Study the drawing (mm; zero at the part's minimum x, y, z) and answer. A direction names the side the tool comes from. Coordinates: 2 decimals unless noted, no trailing zeros. Order: outer loops, then holes, each group sorted by start corner. A loop starts at its lowest first (then second) coordinate and runs counter-clockwise, first axis right, second up.
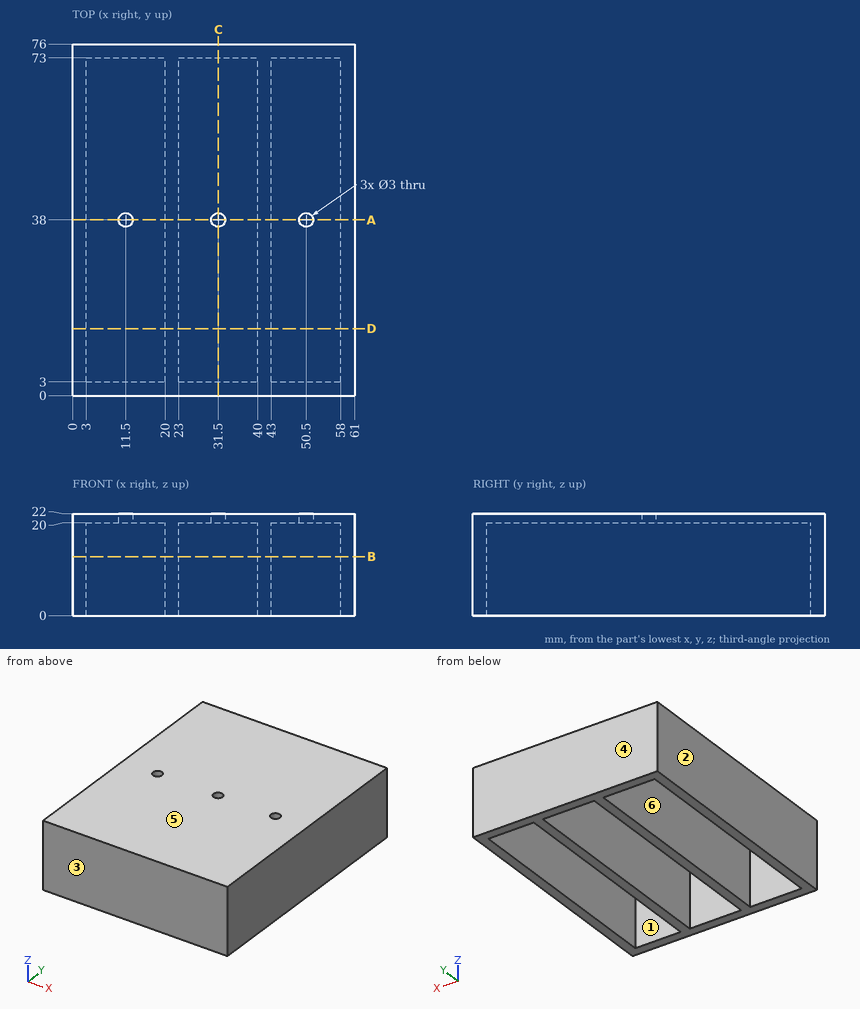
1) Which of the six approach directions +Z, -Z, +X, -X, +Y, -Y give full straight-line access (tool end or side, diameter ignored) to the marked faces 1 and 2?
A:
face 1: -Z
face 2: +Z, -Z, -X, +Y, -Y
2) Determine the mould class of the marked faces 3, 4, 5 and 6 for opening direction Y: pulls with the +Y half, pulls with the -Y half, needs draft (parallel to the pull), parting line crosses it, or undercut.
A:
face 3: pulls with the -Y half
face 4: pulls with the +Y half
face 5: needs draft
face 6: undercut
3) Straight lines are drawn through the part: line 1 (X direction, y = 4.5, z = 1.5); line 2 (Y direction, x = 36.5, z = 14.75); line 3 (Y direction, x = 31.5, z = 21.2). For each, find the intervals that lie inside material, in ascending order.
A:
line 1: x = 0 to 3, 20 to 23, 40 to 43, 58 to 61
line 2: y = 0 to 3, 73 to 76
line 3: y = 0 to 36.5, 39.5 to 76
4) A cutting plane is placed at B-B, the plane z = 12.75. Determine the outline of the cut face in (x, y).
A:
outline: (0, 0) - (61, 0) - (61, 76) - (0, 76) - close; hole (3, 3) - (20, 3) - (20, 73) - (3, 73) - close; hole (23, 3) - (40, 3) - (40, 73) - (23, 73) - close; hole (43, 3) - (58, 3) - (58, 73) - (43, 73) - close
5) A cutting plane is placed at D-D, the plane y = 14.5. Determine the outline of the cut face in (x, z).
A:
outline: (0, 0) - (3, 0) - (3, 20) - (20, 20) - (20, 0) - (23, 0) - (23, 20) - (40, 20) - (40, 0) - (43, 0) - (43, 20) - (58, 20) - (58, 0) - (61, 0) - (61, 22) - (0, 22) - close
6) A cutting plane is placed at A-A, the plane y = 38. Determine the outline of the cut face in (x, z), and give its area (3 significant figures).
A:
outline: (0, 0) - (3, 0) - (3, 20) - (10, 20) - (10, 22) - (0, 22) - close; (13, 20) - (20, 20) - (20, 0) - (23, 0) - (23, 20) - (30, 20) - (30, 22) - (13, 22) - close; (33, 20) - (40, 20) - (40, 0) - (43, 0) - (43, 20) - (49, 20) - (49, 22) - (33, 22) - close; (52, 20) - (58, 20) - (58, 0) - (61, 0) - (61, 22) - (52, 22) - close
area: 344 mm2
7) A cutting plane is placed at C-C, the plane x = 31.5. Determine the outline of the cut face in (y, z), and give its area (3 significant figures).
A:
outline: (0, 0) - (3, 0) - (3, 20) - (36.5, 20) - (36.5, 22) - (0, 22) - close; (39.5, 20) - (73, 20) - (73, 0) - (76, 0) - (76, 22) - (39.5, 22) - close
area: 266 mm2
